Build history of the part. All positions in model axes, mm. Give positions to 0.01 mm unless a question says otherwise; leave off trailing zeros. Loops run counter-clockwise (first coordinate to the right, second up) from the corner with the lowest first, then second, coordinate; pieces in that order, holes last. Notation, with made-up numbers: (-29, 83) - (-3, 83) arc R18 cw to (-3, 105) - close; hole circle Ø6 at (-19, 9.5). An arc over 180 degrees is marked (long way). Return JSON: item names as keys, results as strings. Group by question number.
1) Slice it at B-B (y = 17). Count the separate pieces of the cut face and the enclosed holes in it, and give its area (3 significant figures).
2) Slice it at A-A (z = -3.5). List the corners of the cut face in (x, y).
3) Drill centre lines: probe 1 along Z at (x, y) = (-1, 58.5); probe 2 along X at (y, z) = (35.5, -9); probe 3 along X at (y, z) = (4, -17). Where is each one in solid material? Low to high. Write a range as from..to.
4) Drop flat-ended pins along their axis: pin 1 (6 mm diameter, centred on x = -22, z = -1.5, fed in from +Y); pin 2 (6 mm diameter, centred on x = 22, y = 10, fed in from -Z); pin 3 (1.5 mm diameter, centred on x = -1, y = 57, fed in from +Z). Give the stop position or say it passes through.
5) Mould opens along X. For faces 1 (the face through (-9, 64, -1)), 2 (the face through (29.867, 30.031, -20.099)), 3 (the face through (18, 58, -20)) say: released by +X, released by -X, zero draft, split by the parting line, or undercut.
```python
from build123d import *

# Parameters (mm, degrees)
BOSS_EXTRUDE1_OUTLINE_R   = 36
BOSS_EXTRUDE1_OUTLINE_R_2 = 9.75
BOSS_EXTRUDE1_OUTLINE_W   = 16
BOSS_EXTRUDE1_OUTLINE_H   = 68.8
BOSS_EXTRUDE1_DEPTH       = 64
BOSS_EXTRUDE2_START       = 3
SKETCH2_R                 = 36
BOSS_EXTRUDE2_DEPTH       = 3
SKETCH1_2_R               = 9.75
BOSS_EXTRUDE3_DEPTH       = 12
SKETCH4_R                 = 4
CUT_EXTRUDE1_DEPTH        = 52
SKETCH5_R                 = 1.5
CUT_EXTRUDE2_DEPTH        = 20
SKETCH5_3_R               = 2.3
SKETCH5_3_R_2             = 1.5
CUT_EXTRUDE3_DEPTH        = 6
CUT_EXTRUDE4_DEPTH        = 85.148677946
CUT_EXTRUDE4_DEPTH_BACK   = 85.148677946
SKETCH6_R                 = 3.1
CUT_EXTRUDE5_DEPTH        = 85.148677946
FILLET1_R                 = 3
CIRPATTERN1_COUNT         = 2
FILLET1_OF_CIRPATTERN1_R  = 3
BOSS_EXTRUDE4_DEPTH       = 4
SKETCH9_W                 = 16
SKETCH9_H                 = 68.8
CUT_EXTRUDE6_DEPTH        = 2.5


# Read off the part's stored shape, not the designer's step: Boss-Extrude1
with BuildPart() as part:
    # Boss-Extrude1 outline → Boss-Extrude1 (new body)
    with BuildSketch(Plane(origin=(0, 0, 0), x_dir=(1, 0, 0), z_dir=(0, 1, 0))):
        Circle(BOSS_EXTRUDE1_OUTLINE_R)
        with Locations((-24.35, 0)):
            Circle(BOSS_EXTRUDE1_OUTLINE_R_2, mode=Mode.SUBTRACT)
        Rectangle(BOSS_EXTRUDE1_OUTLINE_W, BOSS_EXTRUDE1_OUTLINE_H, mode=Mode.SUBTRACT)
        with Locations((24.35, 0)):
            Circle(BOSS_EXTRUDE1_OUTLINE_R_2, mode=Mode.SUBTRACT)
    extrude(amount=BOSS_EXTRUDE1_DEPTH)

    # Sketch2 → Boss-Extrude2 (add)
    with BuildSketch(Plane.XZ.offset(BOSS_EXTRUDE2_START)):
        with Locations(Location((0, 0, 0), (0, 0, 270))):
            Circle(SKETCH2_R)
    extrude(amount=-BOSS_EXTRUDE2_DEPTH)

    # Sketch1<2> → Boss-Extrude3 (add)
    with BuildSketch(Plane(origin=(0, 0, 0), x_dir=(1, 0, 0), z_dir=(0, 1, 0))):
        with Locations(Location((-24.35, 0, 0), (0, 0, 270))):
            Circle(SKETCH1_2_R)
        with Locations(Location((24.35, 0, 0), (0, 0, 270))):
            Circle(SKETCH1_2_R)
    extrude(amount=BOSS_EXTRUDE3_DEPTH)

    # Sketch4 → Cut-Extrude1 (cut)
    with BuildSketch(Plane(origin=(0, 64, 0), x_dir=(1, 0, 0), z_dir=(0, 1, 0))):
        with Locations((-24.35, 9.75)):
            Circle(SKETCH4_R)
        with Locations((24.35, -9.75)):
            Circle(SKETCH4_R)
    extrude(amount=-CUT_EXTRUDE1_DEPTH, mode=Mode.SUBTRACT)

    # Sketch5 → Cut-Extrude2 (cut)
    with BuildSketch(Plane(origin=(0, 64, 0), x_dir=(1, 0, 0), z_dir=(0, 1, 0))):
        with Locations(Location((-21.667008817, 18.180779107, 0), (0, 0, 270))):
            Circle(SKETCH5_R)
        with Locations(Location((18.180779107, 21.667008817, 0), (0, 0, 270))):
            Circle(SKETCH5_R)
        with Locations(Location((-18.180779107, -21.667008817, 0), (0, 0, 270))):
            Circle(SKETCH5_R)
        with Locations(Location((21.667008817, -18.180779107, 0), (0, 0, 270))):
            Circle(SKETCH5_R)
    extrude(amount=-CUT_EXTRUDE2_DEPTH, mode=Mode.SUBTRACT)

    # Sketch5<3> → Cut-Extrude3 (cut)
    # profile 1 of 4: a face of its own
    with BuildSketch(Plane(origin=(0, 64, 0), x_dir=(1, 0, 0), z_dir=(0, 1, 0))):
        with Locations(Location((-21.667008817, 18.180779107, 0), (0, 0, 270))):
            Circle(SKETCH5_3_R)
        with Locations(Location((-21.667008817, 18.180779107, 0), (0, 0, 270))):
            Circle(SKETCH5_3_R_2, mode=Mode.SUBTRACT)
    # profile 2 of 4: a face of its own
    with BuildSketch(Plane(origin=(0, 64, 0), x_dir=(1, 0, 0), z_dir=(0, 1, 0))):
        with Locations(Location((18.180779107, 21.667008817, 0), (0, 0, 270))):
            Circle(SKETCH5_3_R)
        with Locations(Location((18.180779107, 21.667008817, 0), (0, 0, 270))):
            Circle(SKETCH5_3_R_2, mode=Mode.SUBTRACT)
    # profile 3 of 4: a face of its own
    with BuildSketch(Plane(origin=(0, 64, 0), x_dir=(1, 0, 0), z_dir=(0, 1, 0))):
        with Locations(Location((21.667008817, -18.180779107, 0), (0, 0, 270))):
            Circle(SKETCH5_3_R)
        with Locations(Location((21.667008817, -18.180779107, 0), (0, 0, 270))):
            Circle(SKETCH5_3_R_2, mode=Mode.SUBTRACT)
    # profile 4 of 4: a face of its own
    with BuildSketch(Plane(origin=(0, 64, 0), x_dir=(1, 0, 0), z_dir=(0, 1, 0))):
        with Locations(Location((-18.180779107, -21.667008817, 0), (0, 0, 270))):
            Circle(SKETCH5_3_R)
        with Locations(Location((-18.180779107, -21.667008817, 0), (0, 0, 270))):
            Circle(SKETCH5_3_R_2, mode=Mode.SUBTRACT)
    extrude(amount=-CUT_EXTRUDE3_DEPTH, mode=Mode.SUBTRACT)

    # Sketch6 → Cut-Extrude4 (cut, two sides: drawn at the far end of the back side and taken through both)
    with BuildSketch(Plane(origin=(0, 64, 0), x_dir=(1, 0, 0), z_dir=(0, 1, 0)).offset(-CUT_EXTRUDE4_DEPTH_BACK)):
        with Locations(Location((-24.681724008, -14.25, 0), (0, 0, 270))):
            Circle(SKETCH6_R)
        with Locations(Location((24.681724008, 14.25, 0), (0, 0, 270))):
            Circle(SKETCH6_R)
    extrude(amount=CUT_EXTRUDE4_DEPTH + CUT_EXTRUDE4_DEPTH_BACK, mode=Mode.SUBTRACT)

    # Sketch7 → Cut-Extrude5 (cut, symmetric)
    with BuildSketch(Plane(origin=(0, 64, 0), x_dir=(1, 0, 0), z_dir=(0, 1, 0))):
        with BuildLine():
            ThreePointArc((-25.259780357, 25.650409281), (-17.207293091, 24.574561329), (-15.464146624, 32.509385863))
            ThreePointArc((-15.464146624, 32.509385863), (-20.648751709, 29.489473594), (-25.259780357, 25.650409281))
        make_face()
    cut_extrude5 = extrude(amount=CUT_EXTRUDE5_DEPTH, both=True, mode=Mode.SUBTRACT)

    # Fillet1
    fillet1_edges = [part.edges().sort_by_distance(p)[0] for p in [
        (-25.259780357, 30.5, -25.650409281),
        (-15.464146624, 30.5, -32.509385863),
        (-20.435059552, 38, -8.929487179),
        (-28.264940448, 38, -8.929487179),
        (20.435059552, 38, 8.929487179),
        (28.264940448, 38, 8.929487179),
    ]]
    fillet(fillet1_edges, radius=FILLET1_R)

    # CirPattern1: Cut-Extrude5 ×2 about axis
    cirpattern1_axis = Axis((0, 0, 0), (0, 1, 0))
    for i in range(1, CIRPATTERN1_COUNT):
        add(cut_extrude5.rotate(cirpattern1_axis, i * 360 / CIRPATTERN1_COUNT), mode=Mode.SUBTRACT)

    # Fillet1 of CirPattern1
    fillet1_of_cirpattern1_edges = [part.edges().sort_by_distance(p)[0] for p in [
        (25.259780357, 30.5, 25.650409281),
        (15.464146624, 30.5, 32.509385863),
        (20.435059552, 38, 8.929487179),
        (28.264940448, 38, 8.929487179),
        (-20.435059552, 38, -8.929487179),
        (-28.264940448, 38, -8.929487179),
    ]]
    fillet(fillet1_of_cirpattern1_edges, radius=FILLET1_OF_CIRPATTERN1_R)

    # Sketch8 → Boss-Extrude4 (add)
    with BuildSketch(Plane(origin=(0, 12, 0), x_dir=(1, 0, 0), z_dir=(0, 1, 0))):
        with BuildLine():
            ThreePointArc((20.386907649, -10.292124542), (24.35, -13.75), (28.313092351, -10.292124542))
            ThreePointArc((28.313092351, -10.292124542), (28.752934813, -9.090438977), (29.653550058, -8.181372549))
            ThreePointArc((29.653550058, -8.181372549), (24.35, 9.75), (19.046449942, -8.181372549))
            ThreePointArc((19.046449942, -8.181372549), (19.947065187, -9.090438977), (20.386907649, -10.292124542))
        make_face()
    extrude(amount=BOSS_EXTRUDE4_DEPTH)

    # Sketch9 → Cut-Extrude6 (cut)
    with BuildSketch(Plane(origin=(0, 0, 0), x_dir=(1, 0, 0), z_dir=(0, 1, 0))):
        Rectangle(SKETCH9_W, SKETCH9_H)
    extrude(amount=-CUT_EXTRUDE6_DEPTH, mode=Mode.SUBTRACT)


solid = part.part
```
Results:
{
 "1": {"separate pieces": "1", "enclosed holes": "5", "area": "2,140 mm2"},
 "2": {"outline": "(-35.83, -3) - (35.83, -3) - (35.83, 64) - (33.45, 64) - (33.45, 16) - (15.25, 16) - (15.25, 64) - (8, 64) - (8, -2.5) - (-8, -2.5) - (-8, 64) - (-15.25, 64) - (-15.25, 12) - (-33.45, 12) - (-33.45, 64) - (-35.83, 64) - close"},
 "3": {"probe 1": "-35.99..-34.4, 34.4..35.99", "probe 2": "-34.86..-28.81, -19.89..-8, 8..20.6, 28.1..34.86", "probe 3": "-31.73..-8, 8..23.25, 26.11..31.73"},
 "4": {"pin 1": "y = 12", "pin 2": "z = -30.58", "pin 3": "z = 36"},
 "5": {"face 1": "zero draft", "face 2": "split by the parting line", "face 3": "undercut"}
}
